Geometry: final body of the model. Coordinates: model frame, mm. Give positions to 0.01 mm unless a question says otherwise; leave off trailing zeros. Loops run counter-clockwise (first coordinate to the right, second up) from the corner with the lowest first, then second, coordinate; pieces in that order, holes last.
1. Section B-B, the plane x = 30. Output: boundary loops of the cut face in (y, z), then the cut area to 3 significant figures.
2. Draft query along Y for faces 1 (the face through (-1, 63.5, 9)), 2 (the face through (-1, -63.5, 9)), 3 (the face through (-10.16, 40.84, 9.39)). Return one class per face: +Y half, -Y half, draft (parallel to the pull), parting line (faces both ways), or undercut.
3. Section C-C, the plane z = 4.75. State how many separate pieces and enclosed holes the cut face has, then the cut area to 3 significant figures.
4. Section A-A, the plane y = -28. Output: boundary loops of the cut face in (x, z), then the cut area to 3 significant figures.
5. Material intervals for line 1 along Y through (x, z) = (-29.5, 17.75); line 2 along Y through (x, z) = (26.5, 3); line 3 along X through (y, z) = (-39.5, 18), sorted ascending.
from build123d import *

# Parameters (mm, degrees)
F0_W     = 174.625
F0_H     = 127
F1_DEPTH = 19.05
F3_D     = 20.6248
F5_D     = 5.1054


with BuildPart() as f1:
    # F0 (on Top) → F1 (new body)
    with BuildSketch(Plane.XY):
        Rectangle(F0_W, F0_H)
    extrude(amount=F1_DEPTH)

    # F3 (through all)
    with Locations(Plane.XY.offset(19.05)):
        with Locations((-35.8775, 35.8775), (-35.8775, -35.8775), (35.8775, 35.8775), (35.8775, -35.8775)):
            Hole(F3_D / 2)

    # F5 (through all)
    with Locations(Plane.XY.offset(19.05)):
        with Locations((-8.9802561211, 43.1052293811), (6.7351920908, 39.9621397388), (-43.1052293811, 8.9802561211), (-39.9621397388, -6.7351920908), (-6.7351920908, -39.9621397388), (8.9802561211, -43.1052293811), (43.1052293811, -8.9802561211), (39.9621397388, 6.7351920908)):
            Hole(F5_D / 2)


solid = f1.part
Answers below:
1. outline: (-63.5, 0) - (-44.35, 0) - (-44.35, 19.05) - (-63.5, 19.05) - close; (-27.4, 0) - (27.4, 0) - (27.4, 19.05) - (-27.4, 19.05) - close; (44.35, 0) - (63.5, 0) - (63.5, 19.05) - (44.35, 19.05) - close
1. area: 1,770 mm2
2. face 1: +Y half
2. face 2: -Y half
2. face 3: undercut
3. separate pieces: 1
3. enclosed holes: 12
3. area: 20,700 mm2
4. outline: (-87.31, 0) - (-42.53, 0) - (-42.53, 19.05) - (-87.31, 19.05) - close; (-29.22, 0) - (29.22, 0) - (29.22, 19.05) - (-29.22, 19.05) - close; (42.53, 0) - (87.31, 0) - (87.31, 19.05) - (42.53, 19.05) - close
4. area: 2,820 mm2
5. line 1: y = -63.5 to -43.98, -27.77 to 27.77, 43.98 to 63.5
5. line 2: y = -63.5 to -40.17, -31.59 to 31.59, 40.17 to 63.5
5. line 3: x = -87.31 to -45.53, -26.22 to -9.25, -4.22 to 26.22, 45.53 to 87.31
